Could you check a few things on this model? Use its own coordinates, in mm. A direction names the side the tool comes from. Give positions to 0.01 mm unless a question says otherwise; leave off trailing zeros. Write each loop counter-clockwise with the first axis right and the second up, starting at its lowest first coordinate (ties: lowest second). Pieces come first, ordered by that corner, then holes. Notation, with made-up numbers: M 60.25,-22.75 L 76.25,-22.75 A31 ccw 76.25,14.25 Z; hole C 19,58 d6. An arc over 180 degrees is marked long. Answer as a JSON object with one key per item and string values. Group by question number.
```python
from build123d import *
from OCP.BRepFilletAPI import BRepFilletAPI_MakeChamfer

# Parameters (mm, degrees)
SKETCH1_W           = 294
SKETCH1_H           = 81
SKETCH1_W_2         = 284
SKETCH1_H_2         = 71
BOSS_EXTRUDE1_DEPTH = 79
FILLET1_R           = 2
CHAMFER1_SIZE       = 2
CHAMFER1_SIZE2      = 3.464101615


with BuildPart() as part:
    # Sketch1 → Boss-Extrude1 (new body)
    with BuildSketch(Plane(origin=(0, 0, 0), x_dir=(1, 0, 0), z_dir=(0, 1, 0))):
        Rectangle(SKETCH1_W, SKETCH1_H)
        Rectangle(SKETCH1_W_2, SKETCH1_H_2, mode=Mode.SUBTRACT)
    extrude(amount=BOSS_EXTRUDE1_DEPTH)

    # Fillet1
    fillet1_edges = [part.edges().sort_by_distance(p)[0] for p in [
        (-147, 39.5, -40.5),
        (147, 39.5, -40.5),
        (147, 39.5, 40.5),
        (-147, 39.5, 40.5),
    ]]
    fillet(fillet1_edges, radius=FILLET1_R)

    # Chamfer1: one chamfer whose edges measure the first distance from different faces: ONE call of the kernel's chamfer builder (chamfer() names one face for all edges)
    chamfer1_edges_1 = [part.edges().sort_by_distance(p)[0] for p in [
        (-142, 0, 0),
    ]]
    chamfer1_side_1 = [part.faces().sort_by_distance(p)[0] for p in [
        (-142, 39.5, 0),
    ]]
    chamfer1_edges_2 = [part.edges().sort_by_distance(p)[0] for p in [
        (0, 0, 35.5),
    ]]
    chamfer1_side_2 = [part.faces().sort_by_distance(p)[0] for p in [
        (0, 39.5, 35.5),
    ]]
    chamfer1_edges_3 = [part.edges().sort_by_distance(p)[0] for p in [
        (142, 0, 0),
    ]]
    chamfer1_side_3 = [part.faces().sort_by_distance(p)[0] for p in [
        (142, 39.5, 0),
    ]]
    chamfer1_edges_4 = [part.edges().sort_by_distance(p)[0] for p in [
        (0, 0, -35.5),
    ]]
    chamfer1_side_4 = [part.faces().sort_by_distance(p)[0] for p in [
        (0, 39.5, -35.5),
    ]]
    chamfer1 = BRepFilletAPI_MakeChamfer(part.part.solid().wrapped)
    for e in chamfer1_edges_1:
        chamfer1.Add(CHAMFER1_SIZE, CHAMFER1_SIZE2, e.wrapped, chamfer1_side_1[0].wrapped)  # the first distance lies on this face
    for e in chamfer1_edges_2:
        chamfer1.Add(CHAMFER1_SIZE, CHAMFER1_SIZE2, e.wrapped, chamfer1_side_2[0].wrapped)  # the first distance lies on this face
    for e in chamfer1_edges_3:
        chamfer1.Add(CHAMFER1_SIZE, CHAMFER1_SIZE2, e.wrapped, chamfer1_side_3[0].wrapped)  # the first distance lies on this face
    for e in chamfer1_edges_4:
        chamfer1.Add(CHAMFER1_SIZE, CHAMFER1_SIZE2, e.wrapped, chamfer1_side_4[0].wrapped)  # the first distance lies on this face
    add(Compound.cast(chamfer1.Shape()), mode=Mode.REPLACE)


solid = part.part
```
1) If we section it at B-B, the plane y = 22: List the corners of the cut face in (x, z) for me, plus the area to 3 significant figures.
2) Please list where these lines run through material, in increasing order: line 1 along X through (y, z) = (6.5, 24.5); line 2 along Z through (x, y) = (-27, 66.5); line 3 along Y through (x, z) = (1, 37.5). Write a range as from..to.
3) If we section it at C-C, the plane x = -27: List the corners of the cut face in (y, z) for me, plus the area to 3 significant figures.
4) If we section it at A-A, the plane z = 8.5: List the corners of the cut face in (x, y) for me, plus the area to 3 significant figures.
5) For faces 4 (the flat face through (-2, 40, -35.5)), 5 (the flat face through (-22, 79, 36)), which set-ups out of +Z, -Z, +X, -X, +Y, -Y let a thin tool reach every point of the face, with its end or its side?
6) We'd pull the mould along Z, two halves only. Please class faces 1 (the flat face through (-2, 39, 40.5)), 2 (the flat face through (147, 39, 1)), 3 (the flat face through (-142, 40, 0)): released by +Z, released by -Z, zero draft, split by the parting line, or undercut.
Taken from the geometry:
{
 "1": {"outline": "M -147,-38.5 A2 ccw -145,-40.5 L 145,-40.5 A2 ccw 147,-38.5 L 147,38.5 A2 ccw 145,40.5 L -145,40.5 A2 ccw -147,38.5 Z; hole M -142,-35.5 L 142,-35.5 L 142,35.5 L -142,35.5 Z", "area": "3,650 mm²"},
 "2": {"line 1": "-147..-142, 142..147", "line 2": "-40.5..-35.5, 35.5..40.5", "line 3": "0.85..79"},
 "3": {"outline": "M 0,-40.5 L 79,-40.5 L 79,-35.5 L 2,-35.5 L 0,-38.96 Z; M 0,38.96 L 2,35.5 L 79,35.5 L 79,40.5 L 0,40.5 Z", "area": "783 mm²"},
 "4": {"outline": "M -147,0 L -145.46,0 L -142,2 L -142,79 L -147,79 Z; M 142,2 L 145.46,0 L 147,0 L 147,79 L 142,79 Z", "area": "783 mm²"},
 "5": {"face 4": "+Y, -Y", "face 5": "+Z, -Z, +X, -X, +Y"},
 "6": {"face 1": "released by +Z", "face 2": "zero draft", "face 3": "undercut"}
}
